Geometry: see drawing. Coordinates: mm, zero at the bounding-box minimum. Give positions to 0.01 mm unless a question says otherwise; leave off trailing zeros. Write each loop counter-clockwise with the first axis right and the second up, starting at its lowest first coordinate (ties: lowest second). Pieces come first, ordered by that corner, then holes. Notation, with made-up numbers: (-36, 12) -> (23, 12) arc R23 cw to (23, 36) -> close; hole circle Ø8 at (84, -17.75). An arc over 180 degrees is marked (long way). Answer as a JSON object with one key per item and string values. Group by question number.
Item 1: First-contact query: pin 1 Ø1.6 at (x, z) = (1, 121.5) entering from -Y (3 decimals); pin 2 Ø1.6 at (x, y) = (2, 6.5) entering from +Z (3 decimals); pin 3 Ø1.6 at (x, z) = (1.5, 227.5) entering from -Y (3 decimals). Flat tips, straight axial feed; report the tip coordinate or a pass-through.
Item 2: Ray query, probe 1 along Y at (x, z) = (0.5, 19) (3 decimals); probe 2 along Z at (x, y) = (1.65, 12.5) (3 decimals). Return the intervals inside material, ascending. Write a range as from..to.
Item 3: Section query B-B on y = 62. Return the cut outline in (x, z) (3 decimals).
Item 4: Section query A-A on x = 1.55. Return the cut outline in (y, z) (3 decimals), plus the area to 3 significant figures.
Item 5: Section query C-C on z = 48. Return the cut outline in (x, y) (3 decimals), plus the area to 3 significant figures.
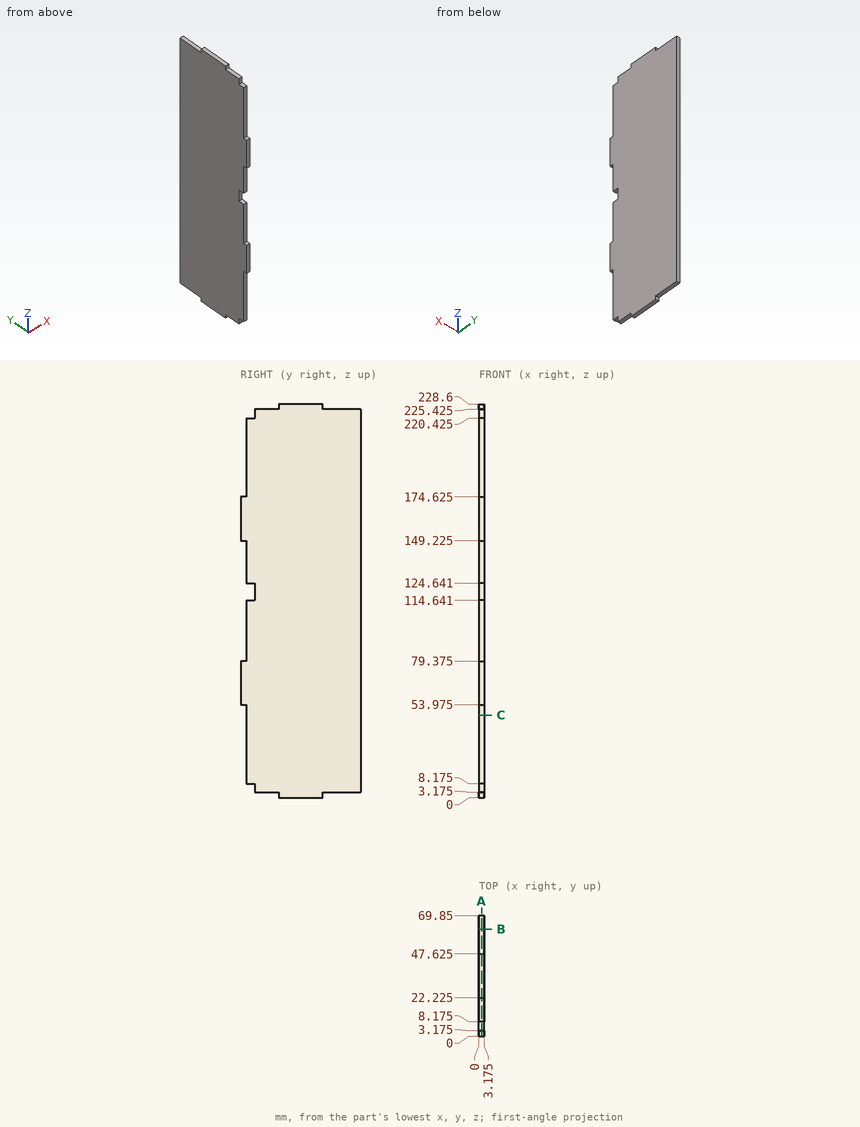
Worked answers:
{
 "1": {"pin 1": "y = 8.175", "pin 2": "z = 220.425", "pin 3": "y = 22.225"},
 "2": {"probe 1": "3.175..69.85", "probe 2": "3.175..225.425"},
 "3": {"outline": "(0, 3.175) -> (3.175, 3.175) -> (3.175, 225.425) -> (0, 225.425) -> close"},
 "4": {"outline": "(0, 53.975) -> (3.175, 53.975) -> (3.175, 8.175) -> (8.175, 8.175) -> (8.175, 3.175) -> (22.225, 3.175) -> (22.225, 0) -> (47.625, 0) -> (47.625, 3.175) -> (69.85, 3.175) -> (69.85, 225.425) -> (47.625, 225.425) -> (47.625, 228.6) -> (22.225, 228.6) -> (22.225, 225.425) -> (8.175, 225.425) -> (8.175, 220.425) -> (3.175, 220.425) -> (3.175, 174.625) -> (0, 174.625) -> (0, 149.225) -> (3.175, 149.225) -> (3.175, 124.641) -> (8.175, 124.641) -> (8.175, 114.641) -> (3.175, 114.641) -> (3.175, 79.375) -> (0, 79.375) -> close", "area": "15,000 mm^2"},
 "5": {"outline": "(0, 3.175) -> (3.175, 3.175) -> (3.175, 69.85) -> (0, 69.85) -> close", "area": "212 mm^2"}
}
